The listing builds one solid part. Answer for the finished solid, in the listing's coordinates (mm). A direction names the side the tool comes from. Round coordinates to 2 decimals unless told otherwise and drop trailing zeros. Order: outer loops, then holes, each group sorted by start corner. A loop starts at its lowest first (then second) coordinate and runs counter-clockwise, first axis right, second up. Notation, with made-up numbers: M 30.5,27.25 L 55.5,27.25 A5 cw 55.5,35.25 Z; hole C 21.5,25 d3. An arc over 180 degrees is marked long. Put each result on its own line as item: value. Start each with the question number.
1. Each of these flat-tipped pins is pushed along its axis until it touches: pin 1 Ø3 at (x, y) = (-34.5, -14) entering from -Z; pin 2 Ø1 at (y, z) = (-2.5, 2.5) entering from +X; pin 3 Ø4.5 at (y, z) = (-4.5, 12) entering from -X. Where does it stop, or does it pass through?
2. The part is cut by section A-A (x = -16). Give the vertices of the cut face in (y, z).
3. Which of the six approach directions +Z, -Z, +X, -X, +Y, -Y give full straight-line access (tool end or side, diameter ignored) to faces 4 (the face through (34, -14, 23.432)), 5 (the face through (-34, -14, 30.544)), 6 (the face through (-34, -12.7, -27)), 7 (the face through (-28.446, -7.727, 51.346))?
4. The mould has two halves that part along X. Classify faces 1 (the face through (-28.486, -7.727, -51.306)), 2 (the face through (-30.986, -7.513, 53.886)), 3 (the face through (34, -12.7, -27)): +X half, -X half, draft (parallel to the pull), parting line (faces both ways), or undercut.
5. The part is cut by section B-B (z = -43). Give the vertices of the cut face in (x, y).
6. Consider line 1 (Z direction, x = -20.5, y = -3.75); line 2 (X direction, y = -5, z = 1.5); line 3 (Z direction, x = 28, y = -11.5). Determine where each line is inside the solid, lowest interval first.
7. The part is cut by section C-C (y = -10.25). Give the vertices of the cut face in (x, z).
from build123d import *

# Parameters (mm, degrees)
F1_DEPTH       = 15.24
F3_DEPTH       = 2.54
F5_D           = 3.2639
F5_CSINK_D     = 6.477
F5_CSINK_ANGLE = 82
F7_DEPTH       = 15.241


with BuildPart() as f1:
    # F0 (on Front) → F1 (new body)
    with BuildSketch(Plane.XZ):
        with BuildLine():
            ThreePointArc((-31.75, -52.07), (-31.0060512242, -53.8660512242), (-29.21, -54.61))
            Line((-29.21, -54.61), (29.21, -54.61))
            ThreePointArc((29.21, -54.61), (31.0060512242, -53.8660512242), (31.75, -52.07))
            Line((31.75, -52.07), (31.75, 52.07))
            ThreePointArc((31.75, 52.07), (31.0060512242, 53.8660512242), (29.21, 54.61))
            Line((29.21, 54.61), (-29.21, 54.61))
            ThreePointArc((-29.21, 54.61), (-31.0060512242, 53.8660512242), (-31.75, 52.07))
            Line((-31.75, 52.07), (-31.75, -52.07))
        make_face()
    extrude(amount=F1_DEPTH)

    # F2 (on face) → F3 (join)
    with BuildSketch(Plane.XZ.offset(15.24)):
        with BuildLine():
            Line((-31.75, 23.4315), (-31.75, 30.5435))
            Line((-31.75, 30.5435), (-35.814, 30.5435))
            ThreePointArc((-35.814, 30.5435), (-38.3284717139, 29.5019717139), (-39.37, 26.9875))
            ThreePointArc((-39.37, 26.9875), (-38.3284717139, 24.4730282861), (-35.814, 23.4315))
            Line((-35.814, 23.4315), (-31.75, 23.4315))
        make_face()
        with BuildLine():
            Line((-31.75, -30.5435), (-31.75, -23.4315))
            Line((-31.75, -23.4315), (-35.814, -23.4315))
            ThreePointArc((-35.814, -23.4315), (-38.3284717139, -24.4730282861), (-39.37, -26.9875))
            ThreePointArc((-39.37, -26.9875), (-38.3284717139, -29.5019717139), (-35.814, -30.5435))
            Line((-35.814, -30.5435), (-31.75, -30.5435))
        make_face()
        with BuildLine():
            Line((35.814, 30.5435), (31.75, 30.5435))
            Line((31.75, 30.5435), (31.75, 23.4315))
            Line((31.75, 23.4315), (35.814, 23.4315))
            ThreePointArc((35.814, 23.4315), (38.3284717139, 24.4730282861), (39.37, 26.9875))
            ThreePointArc((39.37, 26.9875), (38.3284717139, 29.5019717139), (35.814, 30.5435))
        make_face()
        with BuildLine():
            Line((31.75, -23.4315), (31.75, -30.5435))
            Line((31.75, -30.5435), (35.814, -30.5435))
            ThreePointArc((35.814, -30.5435), (38.3284717139, -29.5019717139), (39.37, -26.9875))
            ThreePointArc((39.37, -26.9875), (38.3284717139, -24.4730282861), (35.814, -23.4315))
            Line((35.814, -23.4315), (31.75, -23.4315))
        make_face()
    extrude(amount=-F3_DEPTH)

    # F5 (through all)
    with Locations(Plane.XZ.offset(15.24)):
        with Locations((-35.814, 26.9875), (-35.814, -26.9875), (35.814, 26.9875), (35.814, -26.9875)):
            CounterSinkHole(F5_D / 2, F5_CSINK_D / 2, counter_sink_angle=F5_CSINK_ANGLE)

    # F6 (on face) → F7 (cut, through all)
    with BuildSketch(Plane.XZ.offset(15.24)):
        with BuildLine():
            Line((-26.67, -52.07), (26.67, -52.07))
            ThreePointArc((26.67, -52.07), (28.4660512242, -51.3260512242), (29.21, -49.53))
            Line((29.21, -49.53), (29.21, 49.53))
            ThreePointArc((29.21, 49.53), (28.4660512242, 51.3260512242), (26.67, 52.07))
            Line((26.67, 52.07), (-26.67, 52.07))
            ThreePointArc((-26.67, 52.07), (-28.4660512242, 51.3260512242), (-29.21, 49.53))
            Line((-29.21, 49.53), (-29.21, -49.53))
            ThreePointArc((-29.21, -49.53), (-28.4660512242, -51.3260512242), (-26.67, -52.07))
        make_face()
    extrude(amount=-F7_DEPTH, mode=Mode.SUBTRACT)


solid = f1.part
Resolved:
1. pin 1: z = -30.54
1. pin 2: x = 31.75
1. pin 3: x = -31.75
2. outline: M -15.24,-54.61 L 0,-54.61 L 0,-52.07 L -15.24,-52.07 Z; M -15.24,52.07 L 0,52.07 L 0,54.61 L -15.24,54.61 Z
3. face 4: +X, +Y, -Y
3. face 5: +Z, -X, +Y, -Y
3. face 6: +Z, -Z, -X, +Y
3. face 7: +Y, -Y
4. face 1: undercut
4. face 2: -X half
4. face 3: draft
5. outline: M -31.75,-15.24 L -29.21,-15.24 L -29.21,0 L -31.75,0 Z; M 29.21,-15.24 L 31.75,-15.24 L 31.75,0 L 29.21,0 Z
6. line 1: -54.61 to -52.07, 52.07 to 54.61
6. line 2: -31.75 to -29.21, 29.21 to 31.75
6. line 3: -54.61 to -51.69, 51.69 to 54.61
7. outline: M -31.75,-52.07 A2.54 ccw -29.21,-54.61 L 29.21,-54.61 A2.54 ccw 31.75,-52.07 L 31.75,52.07 A2.54 ccw 29.21,54.61 L -29.21,54.61 A2.54 ccw -31.75,52.07 Z; hole M -29.21,-49.53 A2.54 ccw -26.67,-52.07 L 26.67,-52.07 A2.54 ccw 29.21,-49.53 L 29.21,49.53 A2.54 ccw 26.67,52.07 L -26.67,52.07 A2.54 ccw -29.21,49.53 Z
